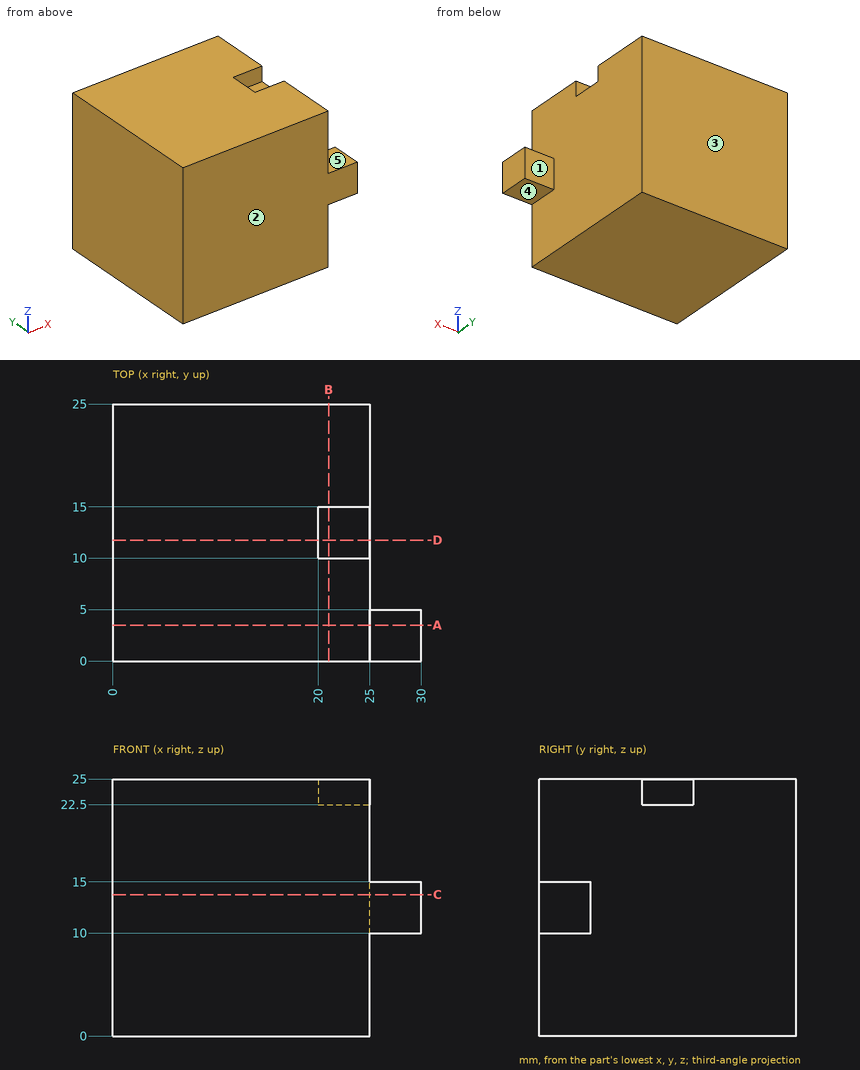
Job drawing, mm, ordinate dimensions from the low corner. One solid piece. A direction names the side the tool comes from. Round coordinates to 2 decimals unless told otherwise and drop trailing zeros. Order: outer loops, then holes, each group sorted by start corner. A loop starts at its lowest first (then second) coordinate and runs counter-clockwise, first axis right, second up. Notation, with made-up numbers: (84, 25.5) -> (123, 25.5) arc R17 ccw to (123, 29.5) -> close; hole circle Ø1 at (75.5, -3.75). An arc over 180 degrees is marked (long way). Write item = value, one per line.
(1) Drill centre lines: L1, parallel to X at y = 14.25, z = 18; L2, parallel to Z at x = 27.5, y = 3.75. Where is each one in solid material? Low to high.
Answers follow:
L1 = 0 to 25
L2 = 10 to 15
(2) 3-axis set-ups, long thin cutter, end or side, ignore diameter. For the marked faces 1, 2, 3, 4 and 5: which of +Z, -Z, +X, -X, +Y, -Y reach the whole face in a straight line?
Answers follow:
face_1 = +Z, -Z, +X, +Y
face_2 = +Z, -Z, +X, -X, -Y
face_3 = +Z, -Z, +X, -X, +Y
face_4 = -Z, +X, +Y, -Y
face_5 = +Z, +X, +Y, -Y
(3) Cut at B-B (x = 21). Write the cut outline in (y, z), plus the area to 4 significant figures.
Answers follow:
outline = (0, 0) -> (25, 0) -> (25, 25) -> (15, 25) -> (15, 22.5) -> (10, 22.5) -> (10, 25) -> (0, 25) -> close
area = 612.5 mm²
(4) Cut at D-D (y = 11.75). Write the cut outline in (x, z), plus the area to 4 significant figures.
Answers follow:
outline = (0, 0) -> (25, 0) -> (25, 22.5) -> (20, 22.5) -> (20, 25) -> (0, 25) -> close
area = 612.5 mm²
(5) Cut at A-A (y = 3.5). Write the cut outline in (x, z), plus the area to 3 significant figures.
Answers follow:
outline = (0, 0) -> (25, 0) -> (25, 10) -> (30, 10) -> (30, 15) -> (25, 15) -> (25, 25) -> (0, 25) -> close
area = 650 mm²
(6) Cut at C-C (z = 13.75). Write the cut outline in (x, y), plus the area to 3 significant figures.
Answers follow:
outline = (0, 0) -> (30, 0) -> (30, 5) -> (25, 5) -> (25, 25) -> (0, 25) -> close
area = 650 mm²
(7) Flat gauge pins, fed straight in: P1, Ø4, axis at x = 28, z = 13, coming from the +Y side; P2, Ø4, axis at x = 3.5, y = 12.5, coming from the -Z side; P3, Ø1.5, axis at x = 22, y = 13.5, coming from the +Z side; P4, Ø4, axis at x = 28.5, y = 1.5, coming from the +Z side. Where does each tip first touch, or does it go through?
Answers follow:
P1 = 5
P2 = 0
P3 = 22.5
P4 = 15
